The listing builds one solid part. Answer for the finished solid, in the listing's coordinates (mm). Give positions to 0.01 mm unless a question says otherwise; leave off trailing zeros. Loops run counter-clockwise (first coordinate to the right, second up) from the corner with the lowest first, then second, coordinate; pieces in that order, holes last. Notation, with made-up numbers: (-5, -29) - (23, -29) arc R17 ccw to (23, 0) - close; hole circle Ø2 at (4.25, -12.75). An arc over 180 degrees is marked (long way). Write each question's results on one line, items separated by ' | '.
from build123d import *

# Parameters (mm, degrees)
SKETCH2_R           = 31.75
SKETCH2_R_2         = 29.294123568
BOSS_EXTRUDE1_DEPTH = 2.794
CUT_EXTRUDE1_DEPTH  = 46.01339384
CUT_EXTRUDE2_DEPTH  = 46.01339384


with BuildPart() as part:
    # Sketch2 → Boss-Extrude1 (new body)
    # profile 1 of 2: a face of its own
    with BuildSketch(Plane(origin=(0, 0, 0), x_dir=(1, 0, 0), z_dir=(0, 1, 0))):
        with Locations(Location((0, 0, 0), (0, 0, 270))):
            Circle(SKETCH2_R)
        Circle(SKETCH2_R_2, mode=Mode.SUBTRACT)
    # profile 2 of 2: a face of its own
    with BuildSketch(Plane(origin=(0, 0, 0), x_dir=(1, 0, 0), z_dir=(0, 1, 0))):
        Circle(SKETCH2_R_2)
    extrude(amount=BOSS_EXTRUDE1_DEPTH)

    # Sketch3 → Cut-Extrude1 (cut, through all)
    with BuildSketch(Plane(origin=(0, 3.175, 0), x_dir=(1, 0, 0), z_dir=(0, 1, 0))):
        with BuildLine():
            Line((5.334, -28.804411461), (5.334, -23.960123568))
            ThreePointArc((5.334, -23.960123568), (0, -18.626123568), (-5.334, -23.960123568))
            Line((-5.334, -23.960123568), (-5.334, -28.804411461))
            ThreePointArc((-5.334, -28.804411461), (0, -29.294123568), (5.334, -28.804411461))
        make_face()
        with BuildLine():
            Line((-20.714073424, -13.170658282), (-24.139502243, -16.596087101))
            ThreePointArc((-24.139502243, -16.596087101), (-20.714073424, -20.714073424), (-16.596087101, -24.139502243))
            Line((-16.596087101, -24.139502243), (-13.170658282, -20.714073424))
            ThreePointArc((-13.170658282, -20.714073424), (-13.170658282, -13.170658282), (-20.714073424, -13.170658282))
        make_face()
        with BuildLine():
            Line((-23.960123568, 5.334), (-28.804411461, 5.334))
            ThreePointArc((-28.804411461, 5.334), (-29.294123568, 0), (-28.804411461, -5.334))
            Line((-28.804411461, -5.334), (-23.960123568, -5.334))
            ThreePointArc((-23.960123568, -5.334), (-18.626123568, 0), (-23.960123568, 5.334))
        make_face()
        with BuildLine():
            Line((-13.170658282, 20.714073424), (-16.596087101, 24.139502243))
            ThreePointArc((-16.596087101, 24.139502243), (-20.714073424, 20.714073424), (-24.139502243, 16.596087101))
            Line((-24.139502243, 16.596087101), (-20.714073424, 13.170658282))
            ThreePointArc((-20.714073424, 13.170658282), (-13.170658282, 13.170658282), (-13.170658282, 20.714073424))
        make_face()
        with BuildLine():
            Line((5.334, 23.960123568), (5.334, 28.804411461))
            ThreePointArc((5.334, 28.804411461), (0, 29.294123568), (-5.334, 28.804411461))
            Line((-5.334, 28.804411461), (-5.334, 23.960123568))
            ThreePointArc((-5.334, 23.960123568), (0, 18.626123568), (5.334, 23.960123568))
        make_face()
        with BuildLine():
            Line((20.714073424, 13.170658282), (24.139502243, 16.596087101))
            ThreePointArc((24.139502243, 16.596087101), (20.714073424, 20.714073424), (16.596087101, 24.139502243))
            Line((16.596087101, 24.139502243), (13.170658282, 20.714073424))
            ThreePointArc((13.170658282, 20.714073424), (13.170658282, 13.170658282), (20.714073424, 13.170658282))
        make_face()
        with BuildLine():
            Line((23.960123568, -5.334), (28.804411461, -5.334))
            ThreePointArc((28.804411461, -5.334), (29.294123568, 0), (28.804411461, 5.334))
            Line((28.804411461, 5.334), (23.960123568, 5.334))
            ThreePointArc((23.960123568, 5.334), (18.626123568, 0), (23.960123568, -5.334))
        make_face()
        with BuildLine():
            Line((13.170658282, -20.714073424), (16.596087101, -24.139502243))
            ThreePointArc((16.596087101, -24.139502243), (20.714073424, -20.714073424), (24.139502243, -16.596087101))
            Line((24.139502243, -16.596087101), (20.714073424, -13.170658282))
            ThreePointArc((20.714073424, -13.170658282), (13.170658282, -13.170658282), (13.170658282, -20.714073424))
        make_face()
    extrude(amount=-CUT_EXTRUDE1_DEPTH, mode=Mode.SUBTRACT)

    # Sketch4 → Cut-Extrude2 (cut, through all)
    with BuildSketch(Plane(origin=(0, 3.175, 0), x_dir=(1, 0, 0), z_dir=(0, 1, 0))):
        with BuildLine():
            Line((-2.413, -1.470474094), (-2.413, 1.470474094))
            ThreePointArc((-2.413, 1.470474094), (2.82575, 0), (-2.413, -1.470474094))
        make_face()
    extrude(amount=-CUT_EXTRUDE2_DEPTH, mode=Mode.SUBTRACT)


solid = part.part
Item 1: A cutting plane is placed at B-B, the plane x = 0. Determine the outline of the cut face in (y, z).
Values found:
outline: (0, -31.75) - (2.79, -31.75) - (2.79, -29.29) - (0, -29.29) - close; (0, -18.63) - (2.79, -18.63) - (2.79, -2.83) - (0, -2.83) - close; (0, 2.83) - (2.79, 2.83) - (2.79, 18.63) - (0, 18.63) - close; (0, 29.29) - (2.79, 29.29) - (2.79, 31.75) - (0, 31.75) - close
Item 2: A cutting plane is placed at C-C, the plane z = 26. Determine the outline of the cut face in (x, y).
Values found:
outline: (-18.22, 0) - (-5.33, 0) - (-5.33, 2.79) - (-18.22, 2.79) - close; (5.33, 0) - (18.22, 0) - (18.22, 2.79) - (5.33, 2.79) - close
Item 3: Find the intervals of material crossed by line 1 along X through (y, z) = (0.8, 0); line 2 along X through (y, z) = (0.65, 17.5); line 3 along X through (y, z) = (2.1, -20), in increasing order. Write a range as [from, to].
Values found:
line 1: x = [-31.75, -29.29], [-18.63, -2.41], [2.83, 18.63], [29.29, 31.75] | line 2: x = [-26.49, -23.49], [-11.64, 11.64], [23.49, 26.49] | line 3: x = [-24.66, -21.4], [-12.57, -3.57], [3.57, 12.57], [21.4, 24.66]
Item 4: A cutting plane is placed at A-A, the plane z = 0. Determine the outline of the cut face in (x, y).
Values found:
outline: (-31.75, 0) - (-29.29, 0) - (-29.29, 2.79) - (-31.75, 2.79) - close; (-18.63, 0) - (-2.41, 0) - (-2.41, 2.79) - (-18.63, 2.79) - close; (2.83, 0) - (18.63, 0) - (18.63, 2.79) - (2.83, 2.79) - close; (29.29, 0) - (31.75, 0) - (31.75, 2.79) - (29.29, 2.79) - close
Item 5: A cutting plane is placed at D-D, the plane x = -27. Determine the outline of the cut face in (y, z), plus the area to 3 significant figures.
Values found:
outline: (0, -16.71) - (2.79, -16.71) - (2.79, -5.33) - (0, -5.33) - close; (0, 5.33) - (2.79, 5.33) - (2.79, 16.71) - (0, 16.71) - close | area: 63.5 mm²
Item 6: For a pull along Z with two mould halves and no side action, classify faces 1 (the face through (-7, 2.794, 0)), 2 (the face through (-30.995, 1.377, -6.883)), 3 (the face through (5.334, 1, 26)) as released by +Z, released by -Z, zero draft, split by the parting line, or undercut.
Values found:
face 1: zero draft | face 2: split by the parting line | face 3: undercut
Item 7: Flat-ended cylindrical pins translate along their axes: P1, Ø1.4, axis at y = 1.5, z = -25.5, coming from the -X side; P2, Ø1.4, axis at x = 25.5, y = 2, coming from the -Z side; P3, Ø1.4, axis at y = 2, z = 27, coming from the +X side. Find the tip coordinate at first contact, or state that the pin passes through.
Values found:
P1: stops at x = -19.82 | P2: stops at z = -19.82 | P3: stops at x = 17.79
